Work out the finished part from the listing and answer in its coordinate system (mm). Face numbers are marked on the shaded views. A direction names the side the tool comes from. Coordinates: 2 decimals unless noted, no trailing zeros. Order: outer loops, then holes, each group sorted by start corner. A loop starts at its lowest first (then second) coordinate and runs counter-clockwise, first axis right, second up. Notation, with made-up numbers: M 31.5,58.5 L 80.5,58.5 A20 ccw 80.5,88.5 Z; hole C -28.75,19 d10. An arc over 180 degrees is marked long. Use a Markdown table: item, result.
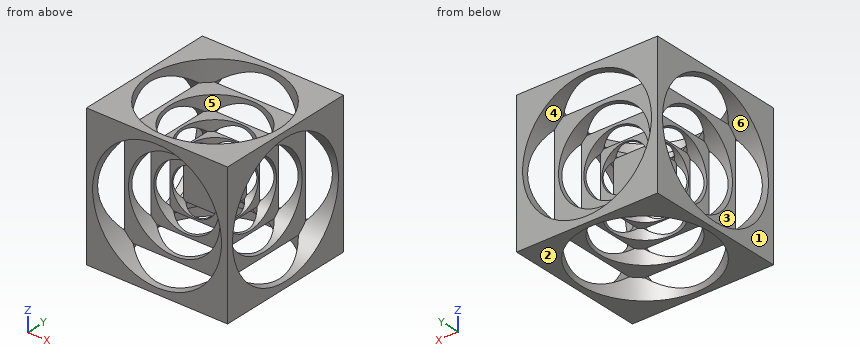
from build123d import *

# Parameters (mm, degrees)
F2_DEPTH = 25


with BuildPart() as f2:
    # F1 (on Front) → F2 (new body, symmetric)
    with BuildSketch(Plane.XZ):
        Polygon((-25, 25), (-25, 0), (-25, -25), (25, -25), (25, 25), align=None)
    extrude(amount=F2_DEPTH, both=True)

    # F3 (on Front) → F4 (revolve, cut)
    with BuildSketch(Plane.XZ):
        Polygon((22.85, 25), (0, 25), (0, 6.1), (8.15, 6.1), (8.15, 8.7), (11.5, 8.7), (11.5, 12.4), (16.2, 12.4), (16.2, 17.6), (22.85, 17.6), align=None)
    revolve(axis=Axis((0, 0, 15.55), (0, 0, 1)), mode=Mode.SUBTRACT)

    # F5 (on Front) → F6 (revolve, cut)
    with BuildSketch(Plane.XZ):
        Polygon((-22.85, -25), (0, -25), (0, -6.1), (-8.15, -6.1), (-8.15, -8.7), (-11.5, -8.7), (-11.5, -12.4), (-16.2, -12.4), (-16.2, -17.6), (-22.85, -17.6), align=None)
    revolve(axis=Axis((0, 0, -15.55), (0, 0, -1)), mode=Mode.SUBTRACT)

    # F7 (on Right) → F8 (revolve, cut)
    with BuildSketch(Plane.YZ):
        Polygon((-25, 22.85), (-25, 0), (-6.1, 0), (-6.1, 8.15), (-8.7, 8.15), (-8.7, 11.5), (-12.4, 11.5), (-12.4, 16.2), (-17.6, 16.2), (-17.6, 22.85), align=None)
    revolve(axis=Axis((0, -15.55, 0), (0, -1, 0)), mode=Mode.SUBTRACT)

    # F9 (on Right) → F10 (revolve, cut)
    with BuildSketch(Plane.YZ):
        Polygon((25, -22.85), (25, 0), (6.1, 0), (6.1, -8.15), (8.7, -8.15), (8.7, -11.5), (12.4, -11.5), (12.4, -16.2), (17.6, -16.2), (17.6, -22.85), align=None)
    revolve(axis=Axis((0, 15.55, 0), (0, 1, 0)), mode=Mode.SUBTRACT)

    # F11 (on Front) → F12 (revolve, cut)
    with BuildSketch(Plane.XZ):
        Polygon((-25.1000002027, 22.85), (-25.1000002027, 0), (-6.2000002027, 0), (-6.2000002027, 8.15), (-8.8000002027, 8.15), (-8.8000002027, 11.5), (-12.5000002027, 11.5), (-12.5000002027, 16.2), (-17.7000002027, 16.2), (-17.7000002027, 22.85), align=None)
    revolve(axis=Axis((-15.6500002027, 0, 0), (-1, 0, 0)), mode=Mode.SUBTRACT)

    # F13 (on Front) → F14 (revolve, cut)
    with BuildSketch(Plane.XZ):
        Polygon((25, -22.85), (25, 0), (6.1, 0), (6.1, -8.15), (8.7, -8.15), (8.7, -11.5), (12.4, -11.5), (12.4, -16.2), (17.6, -16.2), (17.6, -22.85), align=None)
    revolve(axis=Axis((15.55, 0, 0), (1, 0, 0)), mode=Mode.SUBTRACT)


solid = f2.part
(1) A cutting plane is placed at B-B (z = 19.5). Determine the outline of the cut face in (x, y).
Conclusion:
| item | result |
|---|---|
| outline | M -25,-25 L -11.91,-25 L -11.91,-19.5 A22.85 cw -19.5,-11.91 L -25,-11.91 Z; M -25,11.91 L -19.5,11.91 A22.85 cw -11.91,19.5 L -11.91,25 L -25,25 Z; M 11.91,-25 L 25,-25 L 25,-11.91 L 19.5,-11.91 A22.85 cw 11.91,-19.5 Z; M 11.91,19.5 A22.85 cw 19.5,11.91 L 25,11.91 L 25,25 L 11.91,25 Z |
(2) A cutting plane is placed at A-A (x = 22). Determine the outline of the cut face in (y, z).
Conclusion:
| item | result |
|---|---|
| outline | M -25,-25 L -6.17,-25 L -6.17,-22 A22.85 cw -22,-6.17 L -25,-6.17 Z; M -25,6.17 L -22,6.17 A22.85 cw -6.17,22 L -6.17,25 L -25,25 Z; M 6.17,-25 L 25,-25 L 25,-6.17 L 22,-6.17 A22.85 cw 6.17,-22 Z; M 6.17,22 A22.85 cw 22,6.17 L 25,6.17 L 25,25 L 6.17,25 Z |
(3) Determine the mould class of the marked faces 1, 2 and 3 for opening direction Z: pulls with the +Z half, pulls with the -Z half, needs draft (parallel to the pull), parting line crosses it, or undercut.
Conclusion:
| item | result |
|---|---|
| face 1 | needs draft |
| face 2 | pulls with the -Z half |
| face 3 | undercut |
(4) A cutting plane is placed at C-C (y = 0). Give the number of separate pieces and of enclosed holes in the cut face, then the cut area to 3 significant figures.
Conclusion:
| item | result |
|---|---|
| separate pieces | 17 |
| enclosed holes | 0 |
| area | 181 mm2 |
(5) Which of the six approach directions +Z, -Z, +X, -X, +Y, -Y give full straight-line access (tool end or side, diameter ignored) to the marked faces 4, 5 and 6?
Conclusion:
| item | result |
|---|---|
| face 4 | +Y |
| face 5 | +Z |
| face 6 | -X |
(6) Straight lines are drawn through the part: L1, parallel to Z at x = -23, y = 0; L2, parallel to Z at x = 5, y = 16; L3, parallel to Y at x = -6, z = 22.5. For each, find the intervals that lie inside material, in ascending order.
Conclusion:
| item | result |
|---|---|
| L1 | -25 to -22.85, 22.85 to 25 |
| L2 | -17.6 to -15.41, 15.41 to 17.6 |
| L3 | -25 to -22.05, 22.05 to 25 |
(7) Given P1, Ø5, axis at x = 3.5, y = -2.5, coming from the -Z side; P2, Ø10, axis at x = -0.5, z = 1.5, coming from the +Y side; P3, Ø10, axis at y = 9, z = -3, coming from the +X side; P4, Ø1.5, axis at x = 5, y = -18.5, coming from the +Z side, each flat-ended and moving along its own axis, determine where each tip first touches the part or whether it passes through.
Conclusion:
| item | result |
|---|---|
| P1 | z = -6.1 |
| P2 | y = 6.1 |
| P3 | x = 12.4 |
| P4 | through |
